Read the model definition and answer for the solid it produces. Units are mm, in the model's axes. A direction names the side the tool comes from. Coordinates: 2 decimals unless noted, no trailing zeros. Write each loop counter-clockwise with the first axis right and the second up, starting at its lowest first coordinate (ties: lowest second). Pieces come first, ordered by that corner, then holes. Notation, with made-up numbers: (80, 18) -> (128, 18) arc R31 cw to (128, 49) -> close; hole circle Ø9 at (56.25, -36.5). An arc over 180 degrees is marked (long way). One line per item, written item: value. Start each with the question number.
1. Find section D-D, the plane y = -4.5. Write down the section's boundary in (x, z), and give its area (3 significant figures).
2. For faces 5 (the flat face through (0, 8, -3.2)), 6 (the cylindrical face through (-1.22, -2.71, 0.27)), determine the directions among +Z, -Z, +X, -X, +Y, -Y from which every point of the face is accessible in a straight line to the end or side of a thin tool.
3. Find section A-A, the plane x = -1.5. Write down the section's boundary in (y, z).
4. Find section C-C, the plane z = 2. Write down the section's boundary in (x, y), and give its area (3 significant figures).
5. Consider line 1 along Z through (x, y) = (0, 14.25) (3 decimals); line 2 along Y through (x, z) = (-2.25, 1.5); line 3 along X through (y, z) = (14.75, 2.5). Determine where each line is inside the solid, lowest interval first.
6. Given P1, Ø2, axis at y = 9.5, z = -2, coming from the +X side; P2, Ø1, axis at x = -2.5, y = 10, coming from the -Z side; P3, Ø2, axis at y = 12.5, z = 2.5, coming from the +X side, each flat-ended and moving along its own axis, determine where each tip first touches the part or whether it passes through.
7. Find section B-B, the plane y = 6.5. Write down the section's boundary in (x, z).
8. For a pull along Z with two mould halves and no side action, classify faces 1 (the flat face through (2, 0, 0)), 2 (the flat face through (-2.76, 7.89, -1.62)), 3 (the cylindrical face through (1.016, 12.781, 0.133)), 4 (the conical face through (-0.17, 9.14, -0.04)) as pulls with the +Z half, pulls with the -Z half, needs draft (parallel to the pull), parting line crosses it, or undercut.
```python
from build123d import *

# Parameters (mm, degrees)
BOSS_EXTRUDE1_DEPTH     = 16
M2_5_TAPPED_HOLE1_D     = 2.05
M2_5_TAPPED_HOLE1_DEPTH = 6.35
M2_5_TAPPED_HOLE1_TIP   = 0.615882135
SKETCH3_R               = 1.25
BOSS_EXTRUDE2_DEPTH     = 6
CHAMFER1_SIZE           = 0.5


with BuildPart() as part:
    # Sketch1 → Boss-Extrude1 (new body)
    with BuildSketch(Plane(origin=(0, 0, 0), x_dir=(1, 0, 0), z_dir=(0, 1, 0))):
        Polygon((3.695041723, 0), (1.847520861, 3.2), (-1.847520861, 3.2), (-3.695041723, 0), (-1.847520861, -3.2), (1.847520861, -3.2), align=None)
    extrude(amount=BOSS_EXTRUDE1_DEPTH)

    # M2.5 Tapped Hole1
    with Locations(Plane.ZX.offset(16)):
        with Locations((0, 0)):
            Hole(M2_5_TAPPED_HOLE1_D / 2, depth=M2_5_TAPPED_HOLE1_DEPTH)
            with Locations((0, 0, -(M2_5_TAPPED_HOLE1_DEPTH + M2_5_TAPPED_HOLE1_TIP / 2))):  # 118° drill point
                Cone(0, M2_5_TAPPED_HOLE1_D / 2, M2_5_TAPPED_HOLE1_TIP, mode=Mode.SUBTRACT)

    # Sketch3 → Boss-Extrude2 (add)
    with BuildSketch(Plane.XZ):
        with Locations(Location((0, 0, 0), (0, 0, 270))):
            Circle(SKETCH3_R)
    extrude(amount=BOSS_EXTRUDE2_DEPTH)

    # Chamfer1
    chamfer1_edges = [part.edges().sort_by_distance(p)[0] for p in [
        (0, -6, 1.25),
    ]]
    chamfer(chamfer1_edges, length=CHAMFER1_SIZE)


solid = part.part
```
Answer block:
1. outline: circle Ø2.5 at (0, 0)
1. area: 4.91 mm2
2. face 5: -Z, +X, -X, +Y, -Y
2. face 6: -Y
3. outline: (0, -3.2) -> (16, -3.2) -> (16, 3.2) -> (0, 3.2) -> close
4. outline: (-2.54, 0) -> (2.54, 0) -> (2.54, 16) -> (-2.54, 16) -> close
4. area: 81.3 mm2
5. line 1: z = -3.2 to -1.025, 1.025 to 3.2
5. line 2: y = 0 to 16
5. line 3: x = -2.25 to 2.25
6. P1: stops at x = 3.12
6. P2: stops at z = -2.94
6. P3: stops at x = 2.83
7. outline: (-3.7, 0) -> (-1.85, -3.2) -> (1.85, -3.2) -> (3.7, 0) -> (1.85, 3.2) -> (-1.85, 3.2) -> close
8. face 1: needs draft
8. face 2: pulls with the -Z half
8. face 3: undercut
8. face 4: undercut
